Drawing for the job (mm, zero at the part's lowest x, y, z). A direction names the side the tool comes from. Coordinates: 2 decimals unless noted, no trailing zeros. Loops run counter-clockwise (first coordinate to the right, second up) from the corner with the lowest first, then second, coordinate; pieces in that order, holes last. Notation, with made-up numbers: (3, 78) - (31, 78) arc R24 cw to (31, 91) - close; hole circle Ø9 at (40, 24). An arc over 180 degrees is marked (long way). Put each result on its own line as item: value.
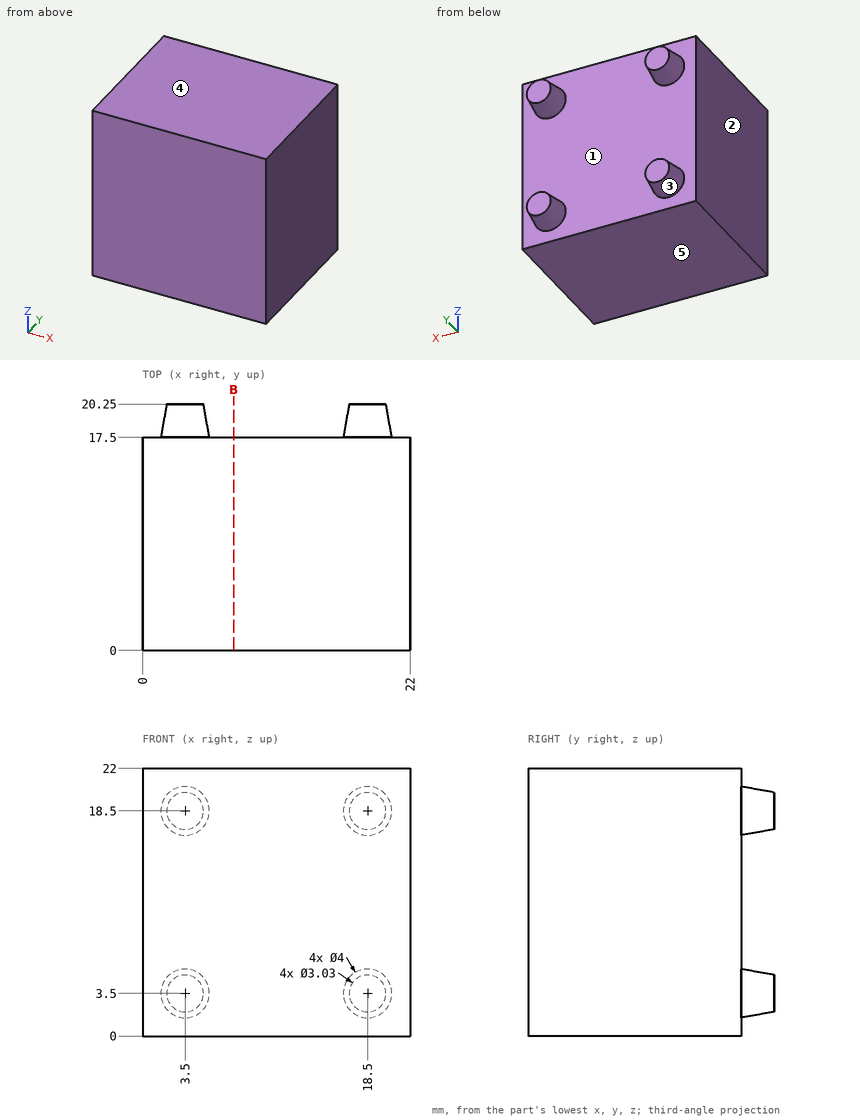
Q1. Wall check: L1, parallel to Y at x = 20.5, z = 16; L2, parallel to Z at x = 17.5, y = 18. Give the ranges that are in metal, low to high. Write a range as from..to.
Determined:
L1: 0..17.5
L2: 1.87..5.13, 16.87..20.13
Q2. Mould opens along Z. For the marked faces 3, 4 and 5 say: +Z half, -Z half, draft (parallel to the pull), parting line (faces both ways), or undercut.
Determined:
face 3: undercut
face 4: +Z half
face 5: -Z half
Q3. Slice it at B-B, the plane x = 7.5. Give the cut face in (y, z).
Determined:
outline: (0, 0) - (17.5, 0) - (17.5, 22) - (0, 22) - close
Q4. Tool access for the marked faces 1 and 2: list every direction of +Z, -Z, +X, -X, +Y, -Y with a clear straight run to the whole face (end or side of a thin tool).
Determined:
face 1: +Y
face 2: +Z, -Z, -X, +Y, -Y
